Input: part model. Units: mm. Frame: model coordinates. A direction names the side the tool comes from. Round coordinates to 2 decimals unless told otherwise and drop trailing zeros. Loops run counter-clockwise (first coordinate to the right, second up) from the corner with the lowest first, then second, coordinate; pieces in that order, holes last. Notation, with made-up numbers: (13, 62) -> (18, 62) arc R24 cw to (18, 95) -> close; hole circle Ø11 at (12, 22.25). An arc over 180 degrees is marked (long way). Answer as a JSON object with one key per item and string values.
```python
from build123d import *

# Parameters (mm, degrees)
SKETCH1_R           = 31
SKETCH1_R_2         = 17
SKETCH1_R_3         = 1.5
BOSS_EXTRUDE1_DEPTH = 4
SKETCH2_R           = 3
CUT_EXTRUDE1_DEPTH  = 1.5
CHAMFER1_SIZE       = 2
CHAMFER1_SIZE2      = 1.154700538


with BuildPart() as part:
    # Sketch1 → Boss-Extrude1 (new body)
    with BuildSketch(Plane(origin=(0, 0, 0), x_dir=(1, 0, 0), z_dir=(0, 1, 0))):
        Circle(SKETCH1_R)
        Circle(SKETCH1_R_2, mode=Mode.SUBTRACT)
        with Locations((0, 24)):
            Circle(SKETCH1_R_3, mode=Mode.SUBTRACT)
        with Locations((20.784609691, 12)):
            Circle(SKETCH1_R_3, mode=Mode.SUBTRACT)
        with Locations((20.784609691, -12)):
            Circle(SKETCH1_R_3, mode=Mode.SUBTRACT)
        with Locations((0, -24)):
            Circle(SKETCH1_R_3, mode=Mode.SUBTRACT)
        with Locations((-20.784609691, -12)):
            Circle(SKETCH1_R_3, mode=Mode.SUBTRACT)
        with Locations((-20.784609691, 12)):
            Circle(SKETCH1_R_3, mode=Mode.SUBTRACT)
    extrude(amount=BOSS_EXTRUDE1_DEPTH)

    # Sketch2 → Cut-Extrude1 (cut)
    with BuildSketch(Plane(origin=(0, 4, 0), x_dir=(1, 0, 0), z_dir=(0, 1, 0))):
        with Locations((0, 24)):
            Circle(SKETCH2_R)
        with Locations((20.784609691, 12)):
            Circle(SKETCH2_R)
        with Locations((20.784609691, -12)):
            Circle(SKETCH2_R)
        with Locations((0, -24)):
            Circle(SKETCH2_R)
        with Locations((-20.784609691, -12)):
            Circle(SKETCH2_R)
        with Locations((-20.784609691, 12)):
            Circle(SKETCH2_R)
    extrude(amount=-CUT_EXTRUDE1_DEPTH, mode=Mode.SUBTRACT)

    # Chamfer1
    chamfer1_edges = [part.edges().sort_by_distance(p)[0] for p in [
        (-31, 4, 0),
    ]]
    chamfer1_side = [part.faces().sort_by_distance(p)[0] for p in [
        (-31, 2, 0),
    ]]
    chamfer(chamfer1_edges, length=CHAMFER1_SIZE, length2=CHAMFER1_SIZE2, reference=chamfer1_side[0])


solid = part.part
```
1) Reachability of faces 5 (the face through (22.2, 1.2, 11.5)), 6 (the face through (17.788, 3.26, 11.868)) from +Z, -Z, +X, -X, +Y, -Y: full face, straight path, thin tool, end or side. Return the list, or none.
Output:
{"face 5": "+Y, -Y", "face 6": "+Y"}
2) Section C-C, the plane y = 0.7. Output: boundary loops of the cut face in (x, z).
Output:
{"outline": "circle Ø62 at (0, 0); hole circle Ø3 at (-20.78, -12); hole circle Ø3 at (-20.78, 12); hole circle Ø34 at (0, 0); hole circle Ø3 at (0, -24); hole circle Ø3 at (0, 24); hole circle Ø3 at (20.78, -12); hole circle Ø3 at (20.78, 12)"}
3) Section A-A, the plane z = 0. Output: boundary loops of the cut face in (x, y).
Output:
{"outline": "(-31, 0) -> (-17, 0) -> (-17, 4) -> (-29.85, 4) -> (-31, 2) -> close; (17, 0) -> (31, 0) -> (31, 2) -> (29.85, 4) -> (17, 4) -> close"}
4) Ray query, probe 1 along Z at (x, y) = (0, 1.05); probe 2 along Z at (x, y) = (22, 1.1); probe 3 along Z at (x, y) = (2, 3.05). Return the intervals inside material, ascending.
Output:
{"probe 1": "z = -31 to -25.5, -22.5 to -17, 17 to 22.5, 25.5 to 31", "probe 2": "z = -21.84 to -12.88, -11.12 to 11.12, 12.88 to 21.84", "probe 3": "z = -30.33 to -26.24, -21.76 to -16.88, 16.88 to 21.76, 26.24 to 30.33"}
5) Section D-D, the plane z = 12. Count the separate pieces of the cut face and the enclosed holes in it, plus the area to 3 significant figures.
Output:
{"separate pieces": "4", "enclosed holes": "0", "area": "96.8 mm^2"}
6) Contact query for flat-ended pins moving along their axis: P1, Ø5, axis at x = 0, z = -24, coming from the +Y side; P2, Ø1.5, axis at y = 0.5, z = -17, coming from the -X side; P3, Ø1, axis at x = -7, y = 3.5, coming from the +Z side. Output: stop coordinate, or through.
Output:
{"P1": "stops at y = 2.5", "P2": "stops at x = -26.4", "P3": "stops at z = 29.63"}
7) Section B-B, the plane x = 0. Output: boundary loops of the cut face in (y, z), plus the area to 3 significant figures.
Output:
{"outline": "(0, -31) -> (2, -31) -> (4, -29.85) -> (4, -27) -> (2.5, -27) -> (2.5, -25.5) -> (0, -25.5) -> close; (0, -22.5) -> (2.5, -22.5) -> (2.5, -21) -> (4, -21) -> (4, -17) -> (0, -17) -> close; (0, 17) -> (4, 17) -> (4, 21) -> (2.5, 21) -> (2.5, 22.5) -> (0, 22.5) -> close; (0, 25.5) -> (2.5, 25.5) -> (2.5, 27) -> (4, 27) -> (4, 29.85) -> (2, 31) -> (0, 31) -> close", "area": "76.7 mm^2"}
8) Draft query along Z for faces 1 (the face through (-4.036, 0.986, -30.736)), 2 (the face through (13, 0, 13)), 3 (the face through (-22.283, 1.232, 11.934)), 4 (the face through (1.3, 2.5, -22.7)). Return one class per face: +Z half, -Z half, draft (parallel to the pull), parting line (faces both ways), or undercut.
Output:
{"face 1": "parting line", "face 2": "draft", "face 3": "undercut", "face 4": "undercut"}
